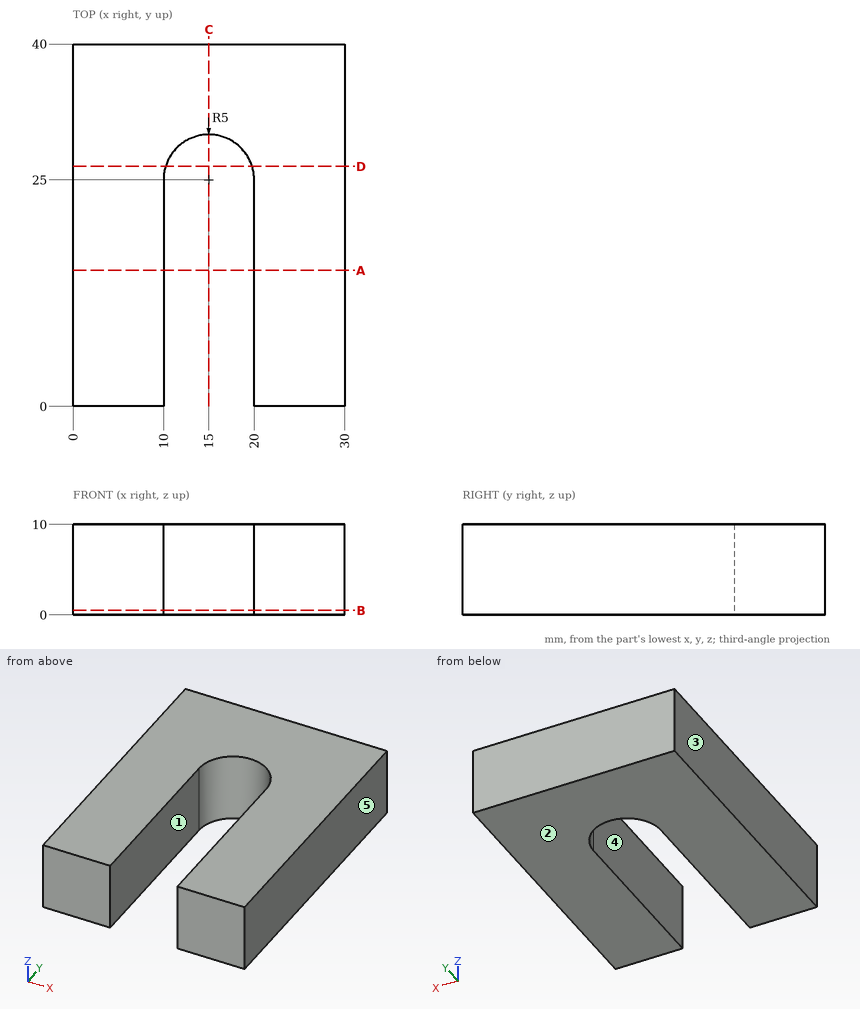
Job drawing, mm, ordinate dimensions from the low corner. One solid piece. A direction names the side the tool comes from. Round coordinates to 2 decimals unless told otherwise and drop trailing zeros. Loops run counter-clockwise (first coordinate to the right, second up) from the corner with the lowest first, then second, coordinate; pieces in that order, holes last. Notation, with made-up numbers: (43.25, -15) -> (84.25, -15) arc R21 cw to (84.25, 16) -> close; hole circle Ø2 at (22.25, 26.5). An arc over 180 degrees is marked (long way). Use CSV: the item, a comma, the result in double quotes. Start each with the question number.
Q1. Mould opens along X. For the marked faces 1, 2 and 3 say: +X half, -X half, draft (parallel to the pull), parting line (faces both ways), or undercut.
Q2. Saw through at B-B on z = 0.5. Give the cut face in (x, y), and give its area (3 significant figures).
Q3. Drill centre lines: L1, parallel to X at y = 21, z = 7.5; L2, parallel to X at y = 28.5, z = 1.5; L3, parallel to Y at x = 10.5, z = 2. Where is each one in solid material? Low to high.
Q4. Saw through at A-A on y = 15. Give the cut face in (x, z), and give its area (3 significant figures).
Q5. Which spindle directions (+Z, -Z, +X, -X, +Y, -Y) get a long thin tool onto all of the face, cutting with end or side? Do the marked faces 4 and 5. Say none if no direction does.
Q6. Saw through at C-C on x = 15. Give the cut face in (y, z), and give its area (3 significant figures).
Q7. Saw through at D-D on y = 26.5. Give the cut face in (x, z), and give its area (3 significant figures).
Solutions:
1,face 1,"undercut"
1,face 2,"draft"
1,face 3,"-X half"
2,outline,"(0, 0) -> (10, 0) -> (10, 25) arc R5 cw to (20, 25) -> (20, 0) -> (30, 0) -> (30, 40) -> (0, 40) -> close"
2,area,"911 mm^2"
3,L1,"x = 0 to 10, 20 to 30"
3,L2,"x = 0 to 11.43, 18.57 to 30"
3,L3,"y = 27.18 to 40"
4,outline,"(0, 0) -> (10, 0) -> (10, 10) -> (0, 10) -> close; (20, 0) -> (30, 0) -> (30, 10) -> (20, 10) -> close"
4,area,"200 mm^2"
5,face 4,"+Z, -Z, -Y"
5,face 5,"+Z, -Z, +X, +Y, -Y"
6,outline,"(30, 0) -> (40, 0) -> (40, 10) -> (30, 10) -> close"
6,area,"100 mm^2"
7,outline,"(0, 0) -> (10.23, 0) -> (10.23, 10) -> (0, 10) -> close; (19.77, 0) -> (30, 0) -> (30, 10) -> (19.77, 10) -> close"
7,area,"205 mm^2"
